For this review, take the finished solid that the model builds, in its own axes (mm). Give positions to 0.01 mm unless a question says otherwise; leave off trailing zeros. Write each loop counter-clockwise with the first axis right and the second up, starting at its lowest first coordinate (ties: lowest second). Pieces come first, ordered by that corner, then holes. Notation, with made-up numbers: M 85.25,29 L 117.25,29 A36 ccw 117.25,64 Z; hole C -2.75,65.5 d7. An arc over 180 degrees is marked long. Answer as a JSON object with one key per item and string values. Group by question number.
```python
from build123d import *

# Parameters (mm, degrees)
SWEEP1_PROFILE_R = 0.254


with BuildPart() as part:
    # Sweep1: sweep along a path in Sketch1
    with BuildLine(Plane(origin=(0, 0, 0), x_dir=(0, 0, -1), z_dir=(1, 0, 0))) as sweep1_path:
        Line((0, 0), (17.54311571, 0))
        ThreePointArc((17.54311571, 0), (17.757805787, -0.047595644), (17.932266287, -0.181463894))
        Line((17.932266287, -0.181463894), (33.38103842, -18.592593586))
        ThreePointArc((33.38103842, -18.592593586), (33.55549892, -18.726461836), (33.770188997, -18.77405748))
        Line((33.770188997, -18.77405748), (40.86001077, -18.77405748))
        ThreePointArc((40.86001077, -18.77405748), (41.11401077, -18.705998385), (41.299951675, -18.52005748))
        Line((41.299951675, -18.52005748), (42.740059095, -16.025718261))
        ThreePointArc((42.740059095, -16.025718261), (42.740059095, -15.517718261), (42.30011819, -15.263718261))
        Line((42.30011819, -15.263718261), (38.1, -15.263718261))
    # Sweep1 profile (on start of the path) → Sweep1 (sweep)
    with BuildSketch(Plane(origin=(0, 0, 0), x_dir=(-1, 0, 0), z_dir=(0, 0, -1))):
        Circle(SWEEP1_PROFILE_R)
    sweep(path=sweep1_path.line)


solid = part.part
```
Item 1: Draft analysis for pull direction Y (two halves, no side actions). For faces 1 (the cylindrical face through (0.055, -9.675, -25.575)), 2 (the cylindrical face through (0.055, -17.379, -42.245)), state which applies: released by +Y, released by -Y, zero draft, split by the parting line, or undercut.
Item 2: To check wall thickness, follow probe 1 along Y at (x, z) = (-0.05, -39); probe 2 along Y at (x, z) = (0.05, -34); probe 3 along Y at (x, z) = (-0.05, -13.5). State the ranges of each line that lie inside material, in increasing order.
Item 3: Consider section A-A (x = 0.15). Give the boundary of the cut face in (y, z).
Item 4: Consider section B-B (z = -5.5). Give the boundary of the cut face in (x, y), plus the area to 3 significant figures.
Result set:
{
 "1": {"face 1": "split by the parting line", "face 2": "undercut"},
 "2": {"probe 1": "y = -19.02 to -18.53, -15.51 to -15.01", "probe 2": "y = -19.02 to -18.53", "probe 3": "y = -0.25 to 0.25"},
 "3": {"outline": "M -18.98,-40.86 A0.71 ccw -18.62,-41.48 L -16.13,-42.92 A0.71 ccw -15.06,-42.3 L -15.06,-38.1 L -15.47,-38.1 L -15.47,-42.3 A0.3 cw -15.92,-42.56 L -18.42,-41.12 A0.3 cw -18.57,-40.86 L -18.57,-33.77 A0.3 cw -18.46,-33.54 L -0.05,-18.09 A0.71 ccw 0.2,-17.54 L 0.2,0 L -0.2,0 L -0.2,-17.54 A0.3 cw -0.31,-17.78 L -18.72,-33.22 A0.71 ccw -18.98,-33.77 Z"},
 "4": {"outline": "C 0,0 d0.51", "area": "0.203 mm^2"}
}
